```python
from build123d import *

# Parameters (mm, degrees)
SKETCH1_W           = 40
SKETCH1_H           = 40
BOSS_EXTRUDE1_DEPTH = 40
SKETCH2_W           = 20
SKETCH2_H           = 20
CUT_EXTRUDE1_DEPTH  = 40
CUT_EXTRUDE2_DEPTH  = 40
SKETCH4_W           = 20
SKETCH4_H           = 20
CUT_EXTRUDE4_DEPTH  = 19.999
CUT_EXTRUDE6_DEPTH  = 19.999
CUT_EXTRUDE7_DEPTH  = 19.999
SKETCH7_W           = 19.9999
SKETCH7_H           = 19.999
CUT_EXTRUDE8_DEPTH  = 19.999
CUT_EXTRUDE9_DEPTH  = 19.999
CUT_EXTRUDE10_DEPTH = 0.0001


with BuildPart() as part:
    # Sketch1 → Boss-Extrude1 (new body)
    with BuildSketch(Plane.XY):
        with Locations((20, 20)):
            Rectangle(SKETCH1_W, SKETCH1_H)
    extrude(amount=BOSS_EXTRUDE1_DEPTH)

    # Sketch2 → Cut-Extrude1 (cut)
    with BuildSketch(Plane.XY.offset(40)):
        with Locations((10, 30)):
            Rectangle(SKETCH2_W, SKETCH2_H)
    extrude(amount=-CUT_EXTRUDE1_DEPTH, mode=Mode.SUBTRACT)

    # Sketch3 → Cut-Extrude2 (cut)
    with BuildSketch(Plane.ZY.offset(-20)):
        Polygon((40, 20), (20, 40), (40, 40), align=None)
    extrude(amount=-CUT_EXTRUDE2_DEPTH, mode=Mode.SUBTRACT)

    # Sketch4 → Cut-Extrude4 (cut)
    with BuildSketch(Plane(origin=(40, 0, 0), x_dir=(0, 0, -1), z_dir=(1, 0, 0))):
        with Locations((-10, 10)):
            Rectangle(SKETCH4_W, SKETCH4_H)
    extrude(amount=-CUT_EXTRUDE4_DEPTH, mode=Mode.SUBTRACT)

    # Sketch5 → Cut-Extrude6 (cut)
    with BuildSketch(Plane(origin=(0, 0, 0), x_dir=(-1, 0, 0), z_dir=(0, 0, -1))):
        Polygon((-39.9999, 39.999), (-20.0001, 20.001), (-39.9999, 20.001), align=None)
    extrude(amount=-CUT_EXTRUDE6_DEPTH, mode=Mode.SUBTRACT)

    # Sketch6 → Cut-Extrude7 (cut)
    with BuildSketch(Plane.ZY.offset(-39.9999)):
        Polygon((0, 20.001), (19.999, 20.001), (20, 39.999), (0, 39.999), align=None)
    extrude(amount=-CUT_EXTRUDE7_DEPTH, mode=Mode.SUBTRACT)

    # Sketch7 → Cut-Extrude8 (cut)
    with BuildSketch(Plane(origin=(0, 20.001, 0), x_dir=(1, 0, 0), z_dir=(0, 1, 0))):
        with Locations((30.00005, -9.9995)):
            Rectangle(SKETCH7_W, SKETCH7_H)
    extrude(amount=-CUT_EXTRUDE8_DEPTH, mode=Mode.SUBTRACT)

    # Sketch8 → Cut-Extrude9 (cut)
    with BuildSketch(Plane.ZY):
        Polygon((0, 0), (20, 20), (0, 20), align=None)
    extrude(amount=-CUT_EXTRUDE9_DEPTH, mode=Mode.SUBTRACT)

    # Sketch9 → Cut-Extrude10 (cut)
    with BuildSketch(Plane.ZY.offset(-20)):
        Polygon((20, 40), (20, 20), (40, 20), align=None)
    extrude(amount=-CUT_EXTRUDE10_DEPTH, mode=Mode.SUBTRACT)


solid = part.part
```
Can you work these out from the model? Positions are in its coordinate system, mm. A direction names the side the tool comes from. Coordinates: 2 decimals unless noted, no trailing zeros. Put each result on its own line as item: value. Start each with the question number.
(1) We'd pull the mould along Z, two halves only. Please class faces 4 (the face through (30, 10, 20)), 5 (the face through (20, 10, 40)), 6 (the face through (20, 30, 10)): +Z half, -Z half, draft (parallel to the pull), parting line (faces both ways), or undercut.
(2) Will these pins go through, and if not, where does the flat tip stop? pin 1 Ø6 at (y, z) = (31, 32.5) entering from -X; pin 2 Ø3 at (x, y) = (14, 14) entering from -Z; pin 3 Ø10 at (y, z) = (9, 11.5) entering from +X.
(3) Which directions (+Z, -Z, +X, -X, +Y, -Y) give clear straight access to the entire face, cutting with the end or side of a thin tool? Please do faces 1 (the face through (30, 30, 10)), 2 (the face through (20, 26, 25)), 3 (the face through (10, 10, 10)).
(4) I need wall thicknesses on probe 1 along Z at (x, y) = (26, 18.5); probe 2 along Y at (x, z) = (12, 35). Which ranges of each line are inside material? Lowest first, please.
Worked answers:
1. face 4: -Z half
1. face 5: +Z half
1. face 6: draft
2. pin 1: stops at x = 20
2. pin 2: stops at z = 12.5
2. pin 3: stops at x = 20
3. face 1: -Z, +X, -Y
3. face 2: +Z, -Z, -X, +Y
3. face 3: -Z, -X, +Y
4. probe 1: z = 20 to 40
4. probe 2: y = 0 to 20
